Verification items for the finished model (mm, model axes). Coordinates: 2 decimals unless noted, no trailing zeros. Write each loop counter-clockwise with the first axis right and the second up, starting at its lowest first coordinate (ties: lowest second). Pieces come first, ordered by that corner, then holes. Notation, with made-up numbers: (87.5, 58) -> (136.5, 58) arc R9 cw to (136.5, 66) -> close; hole circle Ø10 at (61.25, -35.75). An arc over 180 degrees is marked (long way). Answer in a Markdown table with one row per item.
Autodesk Inventor part; units mm, degrees
ref_plane "YZ Plane" through (0, 0, 0) normal (1, 0, 0) x (0, 1, 0)
ref_plane "XZ Plane" through (0, 0, 0) normal (0, 1, 0) x (-1, 0, 0)
ref_plane "XY Plane" through (0, 0, 0) normal (0, 0, 1) x (1, 0, 0)
sketch "Sketch1" plane through (0, 0, 0) normal (1, 0, 0) x (0, 1, 0)
  line L0 (465, 411) -> (465, -123)
  line L1 (465, -123) -> (-15, -123)
  line L2 (-15, -123) -> (-15, 411)
  line L3 (-15, 411) -> (465, 411)
  circle A0 centre (400, -113.5) radius 1.75
  circle A1 centre (50, 401.5) radius 1.75
  circle A2 centre (400, 401.5) radius 1.75
  circle A3 centre (-7.5, -21) radius 1.75
  circle A4 centre (-7.5, 144) radius 1.75
  circle A5 centre (-7.5, 309) radius 1.75
  circle A6 centre (457.5, 144) radius 1.75
  circle A7 centre (457.5, -21) radius 1.75
  circle A8 centre (457.5, 309) radius 1.75
  circle A9 centre (50, -113.5) radius 1.75
  line L4 (47, 380) -> (15, 380)
  line L5 (15, 380) -> (15, 352)
  line L6 (15, 352) -> (47, 352)
  line L7 (47, 352) -> (47, 380)
  circle A10 centre (31, 384) radius 1.6
  circle A11 centre (31, 348) radius 1.6
  line L8 (40.5, 334.5) -> (21.5, 334.5)
  line L9 (21.5, 334.5) -> (21.5, 321.5)
  line L10 (21.5, 321.5) -> (40.5, 321.5)
  line L11 (40.5, 321.5) -> (40.5, 334.5)
  circle A12 centre (63, 292) radius 1.75
  circle A13 centre (63, 12) radius 1.75
  circle A14 centre (63, 62) radius 1.75
  circle A15 centre (38, 37) radius 29.5
  circle A16 centre (13, 292) radius 1.75
  circle A17 centre (63, 242) radius 1.75
  circle A18 centre (13, 12) radius 1.75
  circle A19 centre (13, 62) radius 1.75
  circle A20 centre (13, 242) radius 1.75
  circle A21 centre (38, 267) radius 29.5
  circle A22 centre (25, -23) radius 12.5
  circle A23 centre (37, -73.5) radius 1.25
  circle A24 centre (13, -92.5) radius 1.25
  circle A25 centre (13, -32.5) radius 1.25
  circle A26 centre (25, -53) radius 12.5
  circle A27 centre (13, -62.5) radius 1.25
  circle A28 centre (37, -13.5) radius 1.25
  circle A29 centre (37, -43.5) radius 1.25
  circle A30 centre (25, -83) radius 12.5
  circle A31 centre (265, 270.25) radius 1.6
  circle A32 centre (240, 295.25) radius 1.6
  circle A33 centre (265, -7.25) radius 1.6
  circle A34 centre (240, -7.25) radius 1.6
  circle A35 centre (240, 17.75) radius 1.6
  circle A36 centre (265, 17.75) radius 1.6
  circle A37 centre (265, 295.25) radius 1.6
  circle A38 centre (240, 270.25) radius 1.6
  arc A39 (408.5, -76.2501) -> (408.5, -79.7501) centre (408.5, -78.0001) ccw
  arc A40 (415.5, -89.7501) -> (415.5, -86.2501) centre (415.5, -88.0001) ccw
  arc A41 (408.5, -86.2501) -> (408.5, -89.7501) centre (408.5, -88.0001) ccw
  arc A42 (415.5, -79.7501) -> (415.5, -76.2501) centre (415.5, -78.0001) ccw
  line L12 (408.5, -89.7501) -> (415.5, -89.7501)
  line L13 (415.5, -86.2501) -> (408.5, -86.2501)
  line L14 (408.5, -79.7501) -> (415.5, -79.7501)
  line L15 (415.5, -76.2501) -> (408.5, -76.2501)
  point P0 (0, 0)
  point P1 (37, 276.8868)
  point P2 (37, 271.1132)
extrude "Extrusion1" add sketch "Sketch1" along normal blind 2 contours L0 L1 L2 L3 | L7 L6 L5 L4 | A10 | A11 | L11 L10 L9 L8 | A12 | A13 | A14 | A15 | A16 | A17 | A18 | A19 | A20 | A21 | A22 | A23 | A24 | A25 | A26 | A27 | A28 | A29 | A30 | A31 | A32 | A33 | A34 | A35 | A36 | A37 | A38 | L15 A42 L14 A39 | L12 A41 L13 A40
sketch "Sketch2" plane through (0, 0, 0) normal (-1, 0, 0) x (0, 0, 1)
  line L0 (411, -15) -> (-123, -15)
  line L1 (411, 465) -> (411, -15)
  line L2 (-123, 465) -> (411, 465)
  line L3 (-123, -15) -> (-123, 465)
  circle A0 centre (-113.5, 50) radius 1.75
  circle A1 centre (-21, 457.5) radius 1.75
  circle A2 centre (144, 457.5) radius 1.75
  circle A3 centre (309, -7.5) radius 1.75
  circle A4 centre (144, -7.5) radius 1.75
  circle A5 centre (-21, -7.5) radius 1.75
  circle A6 centre (401.5, 400) radius 1.75
  circle A7 centre (401.5, 50) radius 1.75
  circle A8 centre (-113.5, 400) radius 1.75
  circle A9 centre (309, 457.5) radius 1.75
  line L4 (-73, 425) -> (361, 425)
  line L5 (361, 425) -> (361, 92)
  line L6 (361, 92) -> (-73, 92)
  line L7 (-73, 92) -> (-73, 425)
  point P0 (0, 0)
  dimension "d2" = 50
  dimension "d3" = 50
  dimension "d4" = 40
  dimension "d5" = 107
extrude "Extrusion2" cut sketch "Sketch2" against normal blind 2 contours L4 L5 L6 L7
sketch "Sketch3" plane through (0, 0, 0) normal (-1, 0, 0) x (0, 0, 1)
  line L0 (361, 425) -> (361, 92)
  line L1 (361, 92) -> (-73, 92)
  line L2 (-73, 92) -> (-73, 425)
  line L3 (-73, 425) -> (361, 425)
  line L4 (411, -15) -> (-123, -15)
  line L5 (411, 465) -> (411, -15)
  line L6 (-123, 465) -> (411, 465)
  line L7 (-123, -15) -> (-123, 465)
  circle A0 centre (-113.5, 50) radius 1.75
  circle A1 centre (-21, 457.5) radius 1.75
  circle A2 centre (144, 457.5) radius 1.75
  circle A3 centre (309, -7.5) radius 1.75
  circle A4 centre (144, -7.5) radius 1.75
  circle A5 centre (-21, -7.5) radius 1.75
  circle A6 centre (401.5, 400) radius 1.75
  circle A7 centre (401.5, 50) radius 1.75
  circle A8 centre (-113.5, 400) radius 1.75
  circle A9 centre (309, 457.5) radius 1.75
  circle A10 centre (331, 45) radius 11.5
  line L8 (-60.221, 60.412) -> (-3.121, 60.412) construction
  line L9 (-60.221, 22.612) -> (-60.221, 60.412) construction
  line L10 (-3.121, 22.612) -> (-60.221, 22.612) construction
  line L11 (-3.121, 39.012) -> (-3.121, 22.612) construction
  line L12 (-3.121, 50.012) -> (-3.121, 39.012) construction
  line L13 (-3.121, 60.412) -> (-3.121, 50.012) construction
  arc A11 (-4.921, 57.812) -> (-5.721, 58.612) centre (-5.721, 57.812) ccw construction
  line L14 (-4.921, 30.612) -> (-4.921, 57.812) construction
  arc A12 (-5.721, 29.812) -> (-4.921, 30.612) centre (-5.721, 30.612) ccw construction
  line L15 (-57.621, 29.812) -> (-5.721, 29.812) construction
  arc A13 (-58.421, 30.612) -> (-57.621, 29.812) centre (-57.621, 30.612) ccw construction
  line L16 (-58.421, 57.812) -> (-58.421, 30.612) construction
  arc A14 (-57.621, 58.612) -> (-58.421, 57.812) centre (-57.621, 57.812) ccw construction
  line L17 (-5.721, 58.612) -> (-57.621, 58.612) construction
  circle A15 centre (18.046, 27) radius 1.75 construction
  circle A16 centre (18.0461, 44.7969) radius 3.5 construction
  circle A17 centre (18.0461, 44.7969) radius 4.5
  circle A18 centre (18.046, 27) radius 2.5
  line L18 (-61.221, 61.412) -> (-2.121, 61.412)
  line L19 (-2.121, 61.412) -> (-2.121, 21.612)
  line L20 (-2.121, 21.612) -> (-61.221, 21.612)
  line L21 (-61.221, 21.612) -> (-61.221, 61.412)
  circle A19 centre (-65, 62) radius 1.6
  circle A20 centre (-65, 21) radius 1.6
  circle A21 centre (28, 62) radius 1.6
  circle A22 centre (28, 21) radius 1.6
  circle A23 centre (251, 45) radius 12.5
  circle A24 centre (241.5, 57) radius 1.25
  circle A25 centre (260.5, 33) radius 1.25
  circle A26 centre (225.5, 33) radius 1.25
  circle A27 centre (206.5, 57) radius 1.25
  circle A28 centre (216, 45) radius 12.5
  circle A29 centre (68.0461, 45) radius 8
  point P0 (0, 0)
  dimension "d11" = 23
  dimension "d12" = 60
  dimension "d13" = 80
  dimension "d16" = 9
  dimension "d17" = 5
  dimension "d18" = 1
  dimension "d19" = 1
  dimension "d20" = 1
  dimension "d21" = 1
  dimension "d22" = 9.5
  dimension "d23" = 9.5
  dimension "d24" = 12
  dimension "d25" = 12
  dimension "d26" = 25
  dimension "d27" = 2.5
  dimension "d30" = 35
  dimension "d35" = 80
  dimension "d36" = 16
  dimension "d37" = 50
extrude "Extrusion3" cut sketch "Sketch3" against normal through all contours A10 | A17 | A18 | L18 L19 L20 L21 | A19 | A20 | A21 | A22 | A23 | A24 | A25 | A26 | A27 | A28 | A29
equation "\"d3\" = d2"
equation "\"d19\" = d18"
equation "\"d20\" = d19"
equation "\"d21\" = d19"
equation "\"d23\" = d22"
equation "\"d25\" = d24"
properties part number "Front Panel" material "Aluminum 6061"
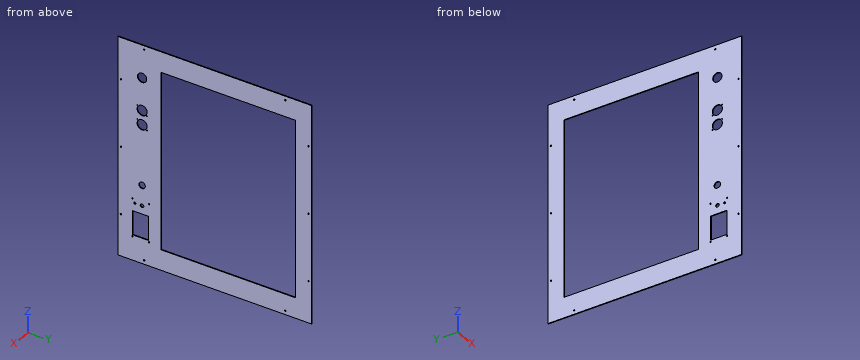
1. Sectioned sample at B-B, the plane z = -41.5. Record the cut outline in (x, y), and give its area (3 significant figures).
Findings below:
| item | result |
|---|---|
| outline | (0, -15) -> (2, -15) -> (2, 21.61) -> (0, 21.61) -> close; (0, 61.41) -> (2, 61.41) -> (2, 92) -> (0, 92) -> close; (0, 425) -> (2, 425) -> (2, 465) -> (0, 465) -> close |
| area | 214 mm² |
2. Sectioned sample at A-A, the plane y = 357.5. Record the cut outline in (x, z), and give its area (3 significant figures).
Findings below:
| item | result |
|---|---|
| outline | (0, -123) -> (2, -123) -> (2, -73) -> (0, -73) -> close; (0, 361) -> (2, 361) -> (2, 411) -> (0, 411) -> close |
| area | 200 mm² |
3. Go/stop test with a flat-tipped pin: pin 1 (5.5 mm diameter, centred on y = 400, z = 401.5, fed in from +X). Record where the tip stops, or that it passes through.
Findings below:
| item | result |
|---|---|
| pin 1 | stops at x = 2 |
4. Sectioned sample at D-D, the plane x = 0.55. Count the separate pieces of the cut face and the enclosed holes in it, and give its area (3 significant figures).
Findings below:
| item | result |
|---|---|
| separate pieces | 1 |
| enclosed holes | 26 |
| area | 108,000 mm² |
5. Sectioned sample at C-C, the plane z = 189. Record the cut outline in (x, y).
Findings below:
| item | result |
|---|---|
| outline | (0, -15) -> (2, -15) -> (2, 92) -> (0, 92) -> close; (0, 425) -> (2, 425) -> (2, 465) -> (0, 465) -> close |
6. Material ranges on probe 1 along Y at (x, z) = (1.45, 28); probe 2 along Y at (x, z) = (0.9, 309); probe 3 along Y at (x, z) = (0.5, 401.5), recorded low to high. Write a range as from..to.
Findings below:
| item | result |
|---|---|
| probe 1 | y = -15..19.4, 22.6..60.4, 63.6..92, 425..465 |
| probe 2 | y = -15..-9.25, -5.75..92, 425..455.75, 459.25..465 |
| probe 3 | y = -15..48.25, 51.75..398.25, 401.75..465 |
